```python
from build123d import *

# Parameters (mm, degrees)
BOSS_EXTRUDE1_DEPTH          = 18.796
CUT_EXTRUDE1_DEPTH           = 67.813105541
CUT_EXTRUDE2_DEPTH           = 67.813105541
F_1_8_0_125_DIAMETER_HOLE2_D = 3.175
FILLET1_R                    = 3.175
F_1_8_0_125_DIAMETER_HOLE1_D = 3.175
LPATTERN1_COUNT              = 7
LPATTERN1_PITCH              = 6.35
MIRROR1_COPY_1_D             = 3.175
MIRROR1_COPY_2_D             = 3.175
MIRROR1_COPY_3_D             = 3.175
MIRROR1_COPY_4_D             = 3.175
MIRROR1_COPY_5_D             = 3.175
MIRROR1_COPY_6_D             = 3.175


with BuildPart() as part:
    # Sketch1 → Boss-Extrude1 (new, symmetric)
    with BuildSketch(Plane.XY):
        with BuildLine():
            Line((0, 0), (0, 35.052))
            ThreePointArc((0, 35.052), (1.190318041, 37.925681959), (4.064, 39.116))
            Line((4.064, 39.116), (50.8, 39.116))
            Line((50.8, 39.116), (50.8, 37.592))
            Line((50.8, 37.592), (4.064, 37.592))
            ThreePointArc((4.064, 37.592), (2.267948776, 36.848051224), (1.524, 35.052))
            Line((1.524, 35.052), (1.524, 0))
            Line((1.524, 0), (0, 0))
        make_face()
    extrude(amount=BOSS_EXTRUDE1_DEPTH, both=True)

    # Sketch2 → Cut-Extrude1 (cut, through all)
    with BuildSketch(Plane.ZY):
        with BuildLine():
            ThreePointArc((0, 0), (-13.290779059, 5.505220941), (-18.796, 18.796))
            Line((-18.796, 18.796), (-18.796, 0))
            Line((-18.796, 0), (0, 0))
        make_face()
        with BuildLine():
            ThreePointArc((18.796, 18.796), (13.290779059, 5.505220941), (0, 0))
            Line((0, 0), (18.796, 0))
            Line((18.796, 0), (18.796, 18.796))
        make_face()
    extrude(amount=-CUT_EXTRUDE1_DEPTH, mode=Mode.SUBTRACT)

    # Sketch3 → Cut-Extrude2 (cut, through all)
    with BuildSketch(Plane.ZY):
        with BuildLine():
            Line((-6.604, 11.811), (-6.604, 25.781))
            ThreePointArc((-6.604, 25.781), (0, 32.385), (6.604, 25.781))
            Line((6.604, 25.781), (6.604, 11.811))
            ThreePointArc((6.604, 11.811), (0, 5.207), (-6.604, 11.811))
        make_face()
    extrude(amount=-CUT_EXTRUDE2_DEPTH, mode=Mode.SUBTRACT)

    # 1/8 (0.125) Diameter Hole2 (through all)
    with Locations(Plane(origin=(0, 31.884241927, -7.5565), x_dir=(0, 0, -1), z_dir=(-1, 0, 0))):
        with Locations((0, 0), (-15.113, 0), (-22.6695, 13.088241927), (-15.113, 26.176483854), (0, 26.176483854), (7.5565, 13.088241927)):
            Hole(F_1_8_0_125_DIAMETER_HOLE2_D / 2)

    # Fillet1
    fillet1_edges = [part.edges().sort_by_distance(p)[0] for p in [
        (50.8, 38.354, 18.796),
        (50.8, 38.354, -18.796),
    ]]
    fillet(fillet1_edges, radius=FILLET1_R)

    # 1/8 (0.125) Diameter Hole1 (through all)
    with Locations(Plane(origin=(47.625, 39.116, -15.621), x_dir=(0, 0, 1), z_dir=(0, 1, 0))):
        with Locations((0, 0)):
            f_1_8_0_125_diameter_hole1 = Hole(F_1_8_0_125_DIAMETER_HOLE1_D / 2)

    # LPattern1: 1/8 (0.125) Diameter Hole1 ×7
    with Locations(*[(-i * LPATTERN1_PITCH, 0, 0) for i in range(1, LPATTERN1_COUNT)]):
        add(f_1_8_0_125_diameter_hole1, mode=Mode.SUBTRACT)

    # Mirror1: 1/8 (0.125) Diameter Hole1 across plane
    add(f_1_8_0_125_diameter_hole1.mirror(Plane.XY), mode=Mode.SUBTRACT)

    # Mirror1 copy 1 (through all)
    with Locations(Plane(origin=(41.275, 39.116, 15.621), x_dir=(0, 0, -1), z_dir=(0, 1, 0))):
        with Locations((0, 0)):
            Hole(MIRROR1_COPY_1_D / 2)

    # Mirror1 copy 2 (through all)
    with Locations(Plane(origin=(34.925, 39.116, 15.621), x_dir=(0, 0, -1), z_dir=(0, 1, 0))):
        with Locations((0, 0)):
            Hole(MIRROR1_COPY_2_D / 2)

    # Mirror1 copy 3 (through all)
    with Locations(Plane(origin=(28.575, 39.116, 15.621), x_dir=(0, 0, -1), z_dir=(0, 1, 0))):
        with Locations((0, 0)):
            Hole(MIRROR1_COPY_3_D / 2)

    # Mirror1 copy 4 (through all)
    with Locations(Plane(origin=(22.225, 39.116, 15.621), x_dir=(0, 0, -1), z_dir=(0, 1, 0))):
        with Locations((0, 0)):
            Hole(MIRROR1_COPY_4_D / 2)

    # Mirror1 copy 5 (through all)
    with Locations(Plane(origin=(15.875, 39.116, 15.621), x_dir=(0, 0, -1), z_dir=(0, 1, 0))):
        with Locations((0, 0)):
            Hole(MIRROR1_COPY_5_D / 2)

    # Mirror1 copy 6 (through all)
    with Locations(Plane(origin=(9.525, 39.116, 15.621), x_dir=(0, 0, -1), z_dir=(0, 1, 0))):
        with Locations((0, 0)):
            Hole(MIRROR1_COPY_6_D / 2)


solid = part.part
```
The model under review builds one solid part; all positions refer to its coordinate system, in mm. A direction names the side the tool comes from. Round coordinates to 2 decimals unless told otherwise and drop trailing zeros. Order: outer loops, then holes, each group sorted by start corner. A loop starts at its lowest first (then second) coordinate and runs counter-clockwise, first axis right, second up.
(1) For P1, Ø3, axis at y = 24, z = -6.5, coming from the +X side; P2, Ø5, axis at x = 15.875, z = 15.621, coming from the -Y side; P3, Ø1.7, axis at x = 1, y = 17.5, coming from the +Z side, all flat-tipped, find the tip position at first contact; note any pin that passes through.
Working result:
P1: stops at x = 1.52
P2: stops at y = 37.59
P3: stops at z = 18.79
(2) Take a section at C-C, the plane x = 38.5. State the section outline as (y, z) points.
Working result:
outline: (37.59, -18.8) - (39.12, -18.8) - (39.12, 18.8) - (37.59, 18.8) - close
(3) Wall thickness on L1, parallel to X at y = 22, z = 9.5; L2, parallel to Y at x = 48.5, z = 12.5; L3, parallel to Y at x = 3, z = 11: over which ranges is each line inside the solid? List them lowest first.
Working result:
L1: x = 0 to 1.52
L2: y = 37.59 to 39.12
L3: y = 37.36 to 38.97
(4) Tool access review of faces 1 (the face through (48.964, 38.343, 16.474)), 2 (the face through (1, 19, 6.604)): name each direction out of +Z, -Z, +X, -X, +Y, -Y from which nothing blocks a thin tool from reaching the whole face with its end or side.
Working result:
face 1: +Y, -Y
face 2: +X, -X
(5) Take a section at B-B, the plane z = -8.5. State the section outline as (x, y) points, plus the area to 3 significant figures.
Working result:
outline: (0, 2.03) - (1.52, 2.03) - (1.52, 4.43) - (0, 4.43) - close; (0, 6.98) - (1.52, 6.98) - (1.52, 30.61) - (0, 30.61) - close; (0, 33.16) - (1.52, 33.16) - (1.52, 35.05) arc R2.54 cw to (4.06, 37.59) - (50.8, 37.59) - (50.8, 39.12) - (4.06, 39.12) arc R4.06 ccw to (0, 35.05) - close
area: 122 mm2
(6) Mouldability with a two-part tool opening along Y and no side actions: class faces 3 (the face through (14.467, 38.343, -16.354)), 4 (the face through (28, 37.592, 0)), 5 (the face through (0.77, 19.4, 16.58)) as released by +Y, released by -Y, zero draft, split by the parting line, or undercut.
Working result:
face 3: zero draft
face 4: released by -Y
face 5: undercut
(7) Take a section at A-A, the plane y = 24.5. State the section outline as (x, z) points.
Working result:
outline: (0, -18.8) - (1.52, -18.8) - (1.52, -6.6) - (0, -6.6) - close; (0, 6.6) - (1.52, 6.6) - (1.52, 18.8) - (0, 18.8) - close
(8) Take a section at D-D, the plane y = 13.5. State the section outline as (x, z) points.
Working result:
outline: (0, -18.03) - (1.52, -18.03) - (1.52, -6.6) - (0, -6.6) - close; (0, 6.6) - (1.52, 6.6) - (1.52, 18.03) - (0, 18.03) - close
